Could you check a few things on this model? Use its own coordinates, in mm. A direction names the side the tool comes from. Coordinates: 2 decimals unless noted, no trailing zeros. Loops run counter-clockwise (first coordinate to the right, second up) from the corner with the lowest first, then second, coordinate; pieces in that order, holes last.
from build123d import *

# Parameters (mm, degrees)
SKETCH1_W                                           = 200
SKETCH1_H                                           = 40
EXTRUDE1_DEPTH                                      = 16
SKETCH2_W                                           = 75
SKETCH2_H                                           = 40
EXTRUDE2_DEPTH                                      = 0.5
M6_TAPPED_HOLE1_D                                   = 5
CBORE_FOR_M6_HEX_SOCKET_HEAD_CAP_SCREW1_D           = 6.6
CBORE_FOR_M6_HEX_SOCKET_HEAD_CAP_SCREW1_CBORE_D     = 11
CBORE_FOR_M6_HEX_SOCKET_HEAD_CAP_SCREW1_CBORE_DEPTH = 6.4


with BuildPart() as part:
    # Sketch1 → Extrude1 (new body)
    with BuildSketch(Plane.XY):
        Rectangle(SKETCH1_W, SKETCH1_H)
    extrude(amount=EXTRUDE1_DEPTH)

    # Sketch2 → Extrude2 (cut)
    with BuildSketch(Plane(origin=(0, 0, 16), x_dir=(-1, 0, 0), z_dir=(0, 0, -1))):
        Rectangle(SKETCH2_W, SKETCH2_H)
    extrude(amount=EXTRUDE2_DEPTH, mode=Mode.SUBTRACT)

    # M6 Tapped Hole1 (through all)
    with Locations(Plane.XY.offset(15.5)):
        with Locations((-23, -10), (23, -10)):
            Hole(M6_TAPPED_HOLE1_D / 2)

    # CBORE for M6 Hex Socket Head Cap Screw1 (through all)
    with Locations(Plane(origin=(0, 0, 0), x_dir=(-1, 0, 0), z_dir=(0, 0, -1))):
        with Locations((-80, 0), (80, 0)):
            CounterBoreHole(CBORE_FOR_M6_HEX_SOCKET_HEAD_CAP_SCREW1_D / 2, CBORE_FOR_M6_HEX_SOCKET_HEAD_CAP_SCREW1_CBORE_D / 2, CBORE_FOR_M6_HEX_SOCKET_HEAD_CAP_SCREW1_CBORE_DEPTH)


solid = part.part
1) For faces 1 (the flat face through (76, 0, 6.4)), 2 (the flat face through (1, 0, 15.5)), 3 (the flat face through (-1, 0, 0)), which set-ups out of +Z, -Z, +X, -X, +Y, -Y let a thin tool reach every point of the face, with its end or its side?
2) If I drill on L1, parallel to X at y = 0.5, z = 8; L2, parallel to Y at x = 80, z = 4.5; L3, parallel to X at y = -3, z = 12.5, over which ranges is the centre line in solid material (lowest first)?
3) Imagine slicing it at A-A on x = -23. List the corners of the cut face in (y, z) for me, plus the area to 4 significant figures.
4) Imagine slicing it at C-C on z = 4.75. List the corners of the cut face in (x, y) for me.
5) Imagine slicing it at B-B on y = -10. List the corners of the cut face in (x, z) for me.
6) Imagine slicing it at D-D on x = -80. List the corners of the cut face in (y, z) for me.
7) Will these pins go through, and if not, where does the flat tip stop? pin 1 (3.5 mm diameter, centred on x = -79, y = 0.5, fed in from -Z); pin 2 (8.5 mm diameter, centred on x = -80, y = 0, fed in from -Z).
8) We'd pull the mould along Y, two halves only. Please class faces 4 (the cylindrical face through (-74.505, 0.242, 3.155)), 5 (the flat face through (-1, 20, 8)), 6 (the flat face through (-100, 0, 8)): released by +Y, released by -Y, zero draft, split by the parting line, or undercut.
Solved:
1. face 1: -Z
1. face 2: +Z, +Y, -Y
1. face 3: -Z, +X, -X, +Y, -Y
2. L1: x = -100 to -83.26, -76.74 to 76.74, 83.26 to 100
2. L2: y = -20 to -5.5, 5.5 to 20
2. L3: x = -100 to -81.37, -78.63 to 78.63, 81.37 to 100
3. outline: (-20, 0) - (-12.5, 0) - (-12.5, 15.5) - (-20, 15.5) - close; (-7.5, 0) - (20, 0) - (20, 15.5) - (-7.5, 15.5) - close
3. area: 542.5 mm2
4. outline: (-100, -20) - (100, -20) - (100, 20) - (-100, 20) - close; hole circle Ø11 at (-80, 0); hole circle Ø5 at (-23, -10); hole circle Ø5 at (23, -10); hole circle Ø11 at (80, 0)
5. outline: (-100, 0) - (-25.5, 0) - (-25.5, 15.5) - (-37.5, 15.5) - (-37.5, 16) - (-100, 16) - close; (-20.5, 0) - (20.5, 0) - (20.5, 15.5) - (-20.5, 15.5) - close; (25.5, 0) - (100, 0) - (100, 16) - (37.5, 16) - (37.5, 15.5) - (25.5, 15.5) - close
6. outline: (-20, 0) - (-5.5, 0) - (-5.5, 6.4) - (-3.3, 6.4) - (-3.3, 16) - (-20, 16) - close; (3.3, 6.4) - (5.5, 6.4) - (5.5, 0) - (20, 0) - (20, 16) - (3.3, 16) - close
7. pin 1: passes through
7. pin 2: stops at z = 6.4
8. face 4: undercut
8. face 5: released by +Y
8. face 6: zero draft
